Read the model definition and answer for the solid it produces. Units are mm, in the model's axes. A direction names the side the tool comes from. Round coordinates to 2 decimals unless told otherwise and drop trailing zeros. Write each loop counter-clockwise with the first axis right and the second up, starting at its lowest first coordinate (ties: lowest second). Pieces come first, ordered by that corner, then holes.
Autodesk Inventor part; units mm, degrees
ref_plane "YZ Plane" through (0, 0, 0) normal (1, 0, 0) x (0, 1, 0)
ref_plane "XZ Plane" through (0, 0, 0) normal (0, 1, 0) x (-1, 0, 0)
ref_plane "XY Plane" through (0, 0, 0) normal (0, 0, 1) x (1, 0, 0)
sketch "Sketch1" plane through (0, 0, 0) normal (0, 1, 0) x (-1, 0, 0)
  line L0 (0, 0) -> (0, 0)
  line L1 (0, -2) -> (0, -23)
  line L2 (0, -25) -> (-1.1394, -25)
  line L3 (-3, -16) -> (-3, -9)
  line L4 (-2, 0) -> (-16, 0)
  line L5 (-18, -2) -> (-18, -2)
  line L6 (-16, -4) -> (-8, -4)
  line L7 (-2, -25) -> (-16, -25)
  line L8 (-18, -23) -> (-18, -23)
  line L9 (-16, -21) -> (-8, -21)
  arc A0 (-3, -9) -> (-8, -4) centre (-8, -9) ccw
  arc A1 (-8, -21) -> (-3, -16) centre (-8, -16) ccw
  arc A2 (-16, 0) -> (-18, -2) centre (-16, -2) ccw
  arc A3 (-18, -2) -> (-16, -4) centre (-16, -2) ccw
  arc A4 (-16, -21) -> (-18, -23) centre (-16, -23) ccw
  arc A5 (-18, -23) -> (-16, -25) centre (-16, -23) ccw
  arc A6 (0, -2) -> (-2, 0) centre (-2, -2) ccw
  arc A7 (-2, -25) -> (0, -23) centre (-2, -23) ccw
  point P0 (-18, -21)
  point P1 (-18, -25)
  point P2 (-16, -2)
  point P3 (-16, -23)
  dimension "d0" = 3
  dimension "d2" = 4
  dimension "d3" = 2
  dimension "d4" = 2
  dimension "d5" = 2
  dimension "d6" = 2
  dimension "d7" = 4
  dimension "d8" = 21
  dimension "d9" = 15
  dimension "d10" = 0
  dimension "d11" = 5
  dimension "d12" = 2
extrude "Extrusion1" add sketch "Sketch1" along normal blind 1.75
sketch "Sketch2" plane through (0, 1.75, 0) normal (0, 1, 0) x (1, 0, 0)
  arc A0 (0, 2) -> (2, 0) centre (2, 2) ccw
  line L0 (0, 23) -> (0, 2)
  arc A1 (2, 25) -> (0, 23) centre (2, 23) ccw
  line L1 (2, 0) -> (2, 25)
  point P0 (0, 0)
extrude "Extrusion2" add sketch "Sketch2" along normal blind 15
hole "Hole1" at (16, 0, -2) at (16, 0, -23) direction (0, 1, 0) diameter 2.4 depth 6.3 tip angle 118
fillet "Fillet1" radius 5 1 edges at (2, 1.75, -12.5)
sketch "Sketch3" plane through (2, 16.75, 0) normal (1, 0, 0) x (0, 0, -1)
  line L0 (2, -2.5) -> (23, -2.5) construction
  line L1 (25, -10) -> (25, 0)
  line L2 (0, -10) -> (0, 0)
  line L3 (0, 0) -> (25, 0)
  point P0 (0, -16.75)
  dimension "d25" = 21
  dimension "d26" = 25
  dimension "d27" = 2
  dimension "d28" = 2.5
hole "Hole2" at (2, 14.25, -2) at (2, 14.25, -23) direction (-1, 0, 0) diameter 1.567 depth 6.3 tip angle 118
sketch "Sketch4" plane through (2, 16.75, 0) normal (1, 0, 0) x (0, 0, -1)
  line L0 (0, 0) -> (25, 0)
  line L1 (4, 0) -> (21, 0)
  line L2 (21, 0) -> (21, -8)
  line L3 (21, -8) -> (4, -8)
  line L4 (4, -8) -> (4, 0)
  line L5 (25, -10) -> (25, 0)
  line L6 (0, -10) -> (0, 0)
  point P0 (0, -16.75)
  dimension "d36" = 8
  dimension "d37" = 25
  dimension "d38" = 4
  dimension "d39" = 4
extrude "Extrusion3" cut sketch "Sketch4" against normal blind 10
fillet "Fillet2" radius 2 2 edges at (1, 8.75, -4) (1, 8.75, -21)
equation "\"d27\" = -0.5 * d25 + 0.5 * d26"
equation "\"d39\" = d38"
properties part number "pi_camera_mount"
Q1. Section C-C (z = -9.75) is taken. Determine the outline of the cut face in (x, y).
Verdict:
outline: (0, 0) - (3, 0) - (3, 3.75) arc R5 cw to (2, 6.75) - (2, 8.75) - (0, 8.75) - close
Q2. Section D-D (y = 14.25) is taken. Determine the outline of the cut face in (x, z).
Verdict:
outline: (0, -22.22) - (2, -22.22) - (2, -21) - (0, -21) - close; (0, -4) - (2, -4) - (2, -2.78) - (0, -2.78) - close; (0.16, -23.78) arc R2 ccw to (2, -25) - (2, -23.78) - close; (0.16, -1.22) - (2, -1.22) - (2, 0) arc R2 ccw to start
Q3. Flat-ended cylindrical pins translate along their axes: pin 1 Ø3 at (x, z) = (16, -23) entering from +Y; pin 2 Ø1 at (y, z) = (3, -4.5) entering from +X; pin 3 Ø4 at (y, z) = (13, -3) entering from +X. Find the tip coordinate at first contact, or state that the pin passes through.
Verdict:
pin 1: stops at y = 1.75
pin 2: stops at x = 4.37
pin 3: stops at x = 2
Q4. Which of the six approach directions +Z, -Z, +X, -X, +Y, -Y give full straight-line access (tool end or side, diameter ignored) to faces 5 (the flat face through (1, 8.75, -13)), 6 (the cylindrical face through (4, 1, -6)), 7 (the flat face through (2, 8, -10)), 8 (the cylindrical face through (0.6, 8.26, -0.57))?
Verdict:
face 5: +X, -X, +Y
face 6: +X, +Y, -Y
face 7: +Z, -Z, +X, +Y
face 8: +Z, -X, +Y, -Y
Q5. Determine the mould class of faces 1 (the flat face through (3, 0, -7)), 2 (the flat face through (12, 1, -4)), 3 (the cylindrical face through (0.986, 14.015, -2.747)), 4 (the flat face through (1, 16.75, -23)) for opening direction Y: pulls with the +Y half, pulls with the -Y half, needs draft (parallel to the pull), parting line crosses it, or undercut.
Verdict:
face 1: pulls with the -Y half
face 2: needs draft
face 3: undercut
face 4: pulls with the +Y half
Q6. Section B-B (y = 10.25) is taken. Determine the outline of the cut face in (x, z).
Verdict:
outline: (0, -23) arc R2 ccw to (2, -25) - (2, -20.94) - (0, -20.94) - close; (0, -4.06) - (2, -4.06) - (2, 0) arc R2 ccw to (0, -2) - close
Q7. Straight lines are drawn through the part: probe 1 along Z at (x, y) = (16, 0.6); probe 2 along Z at (x, y) = (0.85, 14.25); probe 3 along X at (y, z) = (0.75, -2). For each, find the intervals that lie inside material, in ascending order.
Verdict:
probe 1: z = -25 to -24.2, -21.8 to -21, -4 to -3.2, -0.8 to 0
probe 2: z = -24.64 to -23.78, -22.22 to -21, -4 to -2.78, -1.22 to -0.36
probe 3: x = 0 to 14.8, 17.2 to 18
Q8. Section A-A (x = 14.25) is taken. Determine the outline of the cut face in (y, z), then the cut area to 3 significant figures.
Verdict:
outline: (0, -25) - (1.75, -25) - (1.75, -21) - (0, -21) - close; (0, -4) - (1.75, -4) - (1.75, 0) - (0, 0) - close
area: 14.0 mm2
